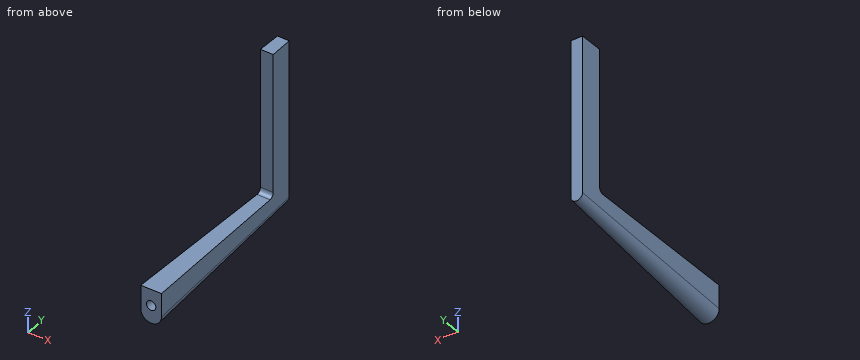
Autodesk Inventor part; units mm, degrees
ref_plane "Work Plane1" through (0, 50.8, 0) normal (0, 1, 0) x (-1, 0, 0)
ref_plane "YZ Plane" through (0, 0, 0) normal (1, 0, 0) x (0, 1, 0)
ref_plane "XY Plane" through (0, 0, 0) normal (0, 0, 1) x (1, 0, 0)
sketch "Sketch6" plane through (0, 0, 0) normal (0, 1, 0) x (-1, 0, 0)
  line L0 (0, 0) -> (5.588, 0)
  line L1 (5.588, 0) -> (5.588, -6.35)
  line L2 (5.588, -6.35) -> (0, -6.35)
  line L3 (0, -6.35) -> (0, 0)
  arc A0 (0, -6.35) -> (5.588, -6.35) centre (2.794, -6.35) ccw
  dimension "d25" = 5.588
  dimension "d26" = 6.35
ref_plane "Work Plane1" through (0, 50.8, 0) normal (0, 1, 0) x (-1, 0, 0)
sketch "Sketch8" plane through (0, 50.8, 0) normal (0, 1, 0) x (-1, 0, 0)
  line L0 (4.3815, 0) -> (1.2065, 0)
  line L1 (1.2065, 0) -> (1.2065, -3.81)
  line L2 (1.2065, -3.81) -> (4.3815, -3.81)
  line L3 (4.3815, -3.81) -> (4.3815, 0)
  arc A0 (1.2065, -3.81) -> (4.3815, -3.81) centre (2.794, -3.81) ccw
  point P0 (0, 0)
  dimension "d27" = 3.175
  dimension "d28" = 3.81
  dimension "d49" = 1.2065
loft "Loft1" add profiles "Sketch6", "Sketch8"
sketch "Sketch9" plane through (-5.588, 0, 0) normal (0, 0, 1) x (1, 0, 0)
  line L0 (0, 0) -> (5.588, 0)
  line L1 (5.588, 0) -> (4.3815, 50.8)
  line L2 (1.2065, 50.8) -> (4.3815, 50.8)
  line L3 (0, 0) -> (1.2065, 50.8)
  line L4 (4.3815, 50.8) -> (5.588, 0)
  line L5 (4.5323, 44.45) -> (1.0557, 44.45)
  line L6 (0, 0) -> (1.2065, 50.8)
  dimension "d34" = 6.35
extrude "Extrusion5" add sketch "Sketch9" along normal blind 38.608 contours L3 L2 L1 L5
sketch "Sketch12" plane through (-2.794, 0, -6.35) normal (0, -1, 0) x (1, 0, 0)
  circle A0 centre (0, 1.9685) radius 1.27
  arc A1 (-2.794, 0) -> (2.794, 0) centre (0, 0) ccw
  line L0 (0, -2.794) -> (0, 1.9685)
  point P0 (2.794, 6.35)
  dimension "d44" = 2.54
  dimension "d46" = 4.7625
extrude "Extrusion8" cut sketch "Sketch12" against normal blind 10.16
fillet "Fillet3" radius 1.27 1 edges at (-2.794, 44.45, 0)
properties part number "RudderStabilizingFins"
The listing builds one solid part. Answer for the finished solid, in the listing's coordinates (mm). Round coordinates to 2 decimals unless told otherwise and drop trailing zeros. Write each loop counter-clockwise with the first axis right and the second up, starting at its lowest first coordinate (ties: lowest second). Pieces come first, ordered by that corner, then holes. Notation, with made-up numbers: M 83.25,87 L 131.25,87 A27 ccw 131.25,108 Z; hole C 76,63.25 d3. An arc over 180 degrees is marked long. Write each question's results on one line, items separated by ' | '. Start each with the question number.
Item 1: Straight lines are drawn through the part: L1, parallel to Y at x = -2.65, z = 20; L2, parallel to Z at x = -2.55, y = 8; L3, parallel to Z at x = -2.75, y = 11.5. For each, find the intervals that lie inside material, in ascending order. Write a range as [from, to].
Item 2: A cutting plane is placed at A-A on z = 2.5. Write down the section's boundary in (x, y).
Item 3: Flat-ended cylindrical pins translate along their axes: pin 1 Ø3 at (x, z) = (-1, 20) entering from -Y; pin 2 Ø2 at (y, z) = (32.5, -3.5) entering from +X; pin 3 Ø6 at (y, z) = (44.5, 32.5) entering from -X; pin 4 Ø1.3 at (x, z) = (-3.5, -4) entering from -Y. Find the tip coordinate at first contact, or state that the pin passes through.
Check sheet entries:
1) L1: [44.45, 50.8] | L2: [-8.54, -5.63], [-3.14, 0] | L3: [-8.3, 0]
2) outline: M -4.53,44.45 L -1.06,44.45 L -1.21,50.8 L -4.38,50.8 Z
3) pin 1: y = 44.45 | pin 2: x = -0.75 | pin 3: x = -4.53 | pin 4: y = 0
